Could you check a few things on this model? Use its own coordinates, in mm. A direction names the side the tool comes from. Give positions to 0.01 mm unless a question says otherwise; leave off trailing zeros. Write each loop counter-clockwise with the first axis right and the second up, starting at its lowest first coordinate (ties: lowest second). Pieces come first, ordered by that corner, then holes. Notation, with made-up numbers: M 86,40.5 L 142,40.5 A25 cw 142,62.5 Z; hole C 17,73.5 d6. An arc over 180 degrees is marked long. Answer as CSV lines item,"result". Start each with the question number.
from build123d import *

# Parameters (mm, degrees)
FILLET_1_R  = 0.2
HEX_2_DEPTH = 1.56


with BuildPart() as part:
    # Эскиз1 → Body (revolve)
    with BuildSketch(Plane.XY):
        with BuildLine():
            Line((0, 2.375), (0, 0))
            Line((0, 0), (8.75, 0))
            Line((8.75, 0), (8.75, 2.055))
            Line((8.75, 2.055), (8.305, 2.5))
            Line((8.305, 2.5), (2.75, 2.5))
            Line((2.75, 2.5), (2.75, 4.75))
            Line((2.75, 4.75), (2.370164642, 4.75))
            ThreePointArc((2.370164642, 4.75), (0.992749859, 3.754440885), (0, 2.375))
        make_face()
    revolve(axis=Axis((-3.643489966, 0, 0), (-1, 0, 0)))

    # Скругление1
    fillet_1_edges = [part.edges().sort_by_distance(p)[0] for p in [
        (2.75, -2.5, 0),
    ]]
    fillet(fillet_1_edges, radius=FILLET_1_R)

    # Эскиз2 → Вырез-Повернуть1 (revolve, cut)
    with BuildSketch(Plane.XY):
        Polygon((0, 0), (0, 1.5), (1.56, 1.5), (2.426025404, 0), align=None)
    revolve(axis=Axis((2.426025404, 0, 0), (-1, 0, 0)), mode=Mode.SUBTRACT)

    # Эскиз3 → Hex 2 (cut)
    with BuildSketch(Plane.ZY):
        Polygon((-1.5, -0.866025404), (0, -1.732050808), (1.5, -0.866025404), (1.5, 0.866025404), (0, 1.732050808), (-1.5, 0.866025404), align=None)
    extrude(amount=-HEX_2_DEPTH, mode=Mode.SUBTRACT)


solid = part.part
1. On a 3-axis mill with a long thin cutter (end or side, diameter ignored), from which of +Z, -Z, +X, -X, +Y, -Y can I reach the whole of each face in a straight line? I mean faces 1 (the flat face through (0.769, 1.305, -0.74)), 2 (the cylindrical face through (5.59, -0.54, 2.44)), 3 (the flat face through (8.75, 0, 0)). Say none if no direction works.
2. Imagine slicing it at A-A, the plane x = 2. Please give me the cut outline in (y, z).
3. Please list where these lines run through material, in increasing order: line 1 (Z direction, x = 1.5, y = -1); line 2 (Y direction, x = 2, z = 0); line 3 (Z direction, x = 2.5, y = -0.25).
4. Thinking about a two-plate mould opening in Z: for faces 4 (the flat face through (1, 0, -1.5)), 5 (the cylindrical face through (2.557, 2.192, 4.214)), 6 (the flat face through (2.75, -2.04, 2.04)), which applies, pulls with the +Z half, pulls with the -Z half, needs draft (parallel to the pull), parting line crosses it, or undercut?
5. Imagine slicing it at B-B, the plane y = -3. Please give me the cut outline in (x, z).
6. Will these pins go through, and if not, where does the flat tip stop? P1, Ø1.7, axis at x = 0.5, y = 0, coming from the -Z side; P2, Ø3, axis at x = 6.5, z = -3, coming from the +Y side; P3, Ø0.5, axis at x = 1, y = 0, coming from the +Z side.
7. Imagine slicing it at C-C, the plane x = 5.75. Please give me the cut outline in (y, z).
Solutions:
1,face 1,"-X"
1,face 2,"+X"
1,face 3,"+Z, -Z, +X, +Y, -Y"
2,outline,"C 0,0 d9.09; hole C 0,0 d1.48"
3,line 1,"-4.08 to -1.27, 1.27 to 4.08"
3,line 2,"-4.55 to -0.74, 0.74 to 4.55"
3,line 3,"-4.74 to 4.74"
4,face 4,"undercut"
4,face 5,"parting line crosses it"
4,face 6,"needs draft"
5,outline,"M 2.37,-3.68 L 2.75,-3.68 L 2.75,3.68 L 2.37,3.68 A4.39 ccw Z"
6,P1,"z = -4.08"
6,P2,"y = 2"
6,P3,"z = 4"
7,outline,"C 0,0 d5"
